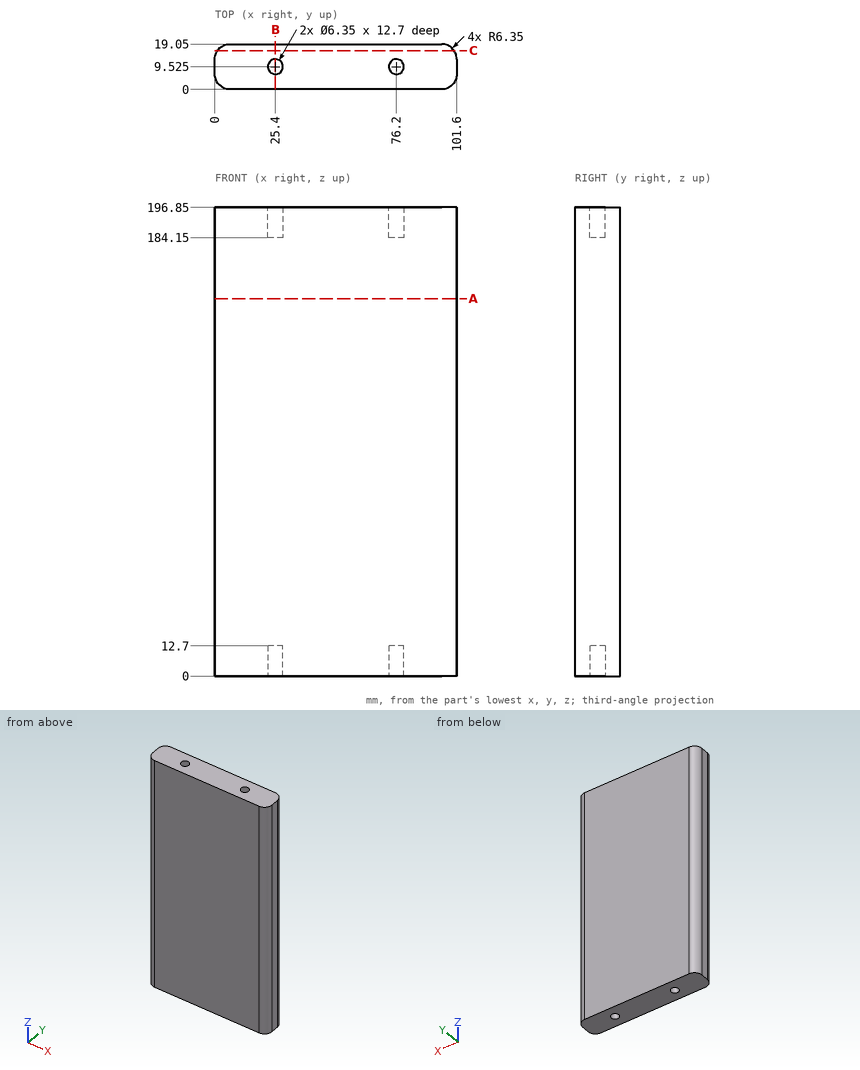
Verification items for this drawing (mm, ordinates from the low corner). Give positions to 0.01 mm unless a question says otherwise; leave off trailing zeros. Write each loop counter-clockwise with the first axis right and the second up, starting at its lowest first coordinate (ties: lowest second). Pieces come first, ordered by that corner, then holes. Notation, with made-up numbers: (-40, 69.5) - (2, 69.5) arc R24 ccw to (2, 91.5) - close; hole circle Ø8 at (51.25, 53). An arc over 180 degrees is marked (long way). Answer as a JSON object with one key per item and string values. Group by question number.
1) Depth check by flat-ended pin: P1, Ø5, axis at x = 76.2, y = 9.525, coming from the +Z side; P2, Ø1.5, axis at y = 15, z = 123, coming from the +X side; P3, Ø3, axis at y = 2.5, z = 138.5, coming from the -X side. Enter the tip coordinate at first touch or a pass-through.
2) Sectioned sample at C-C (y = 16.25). Record the cut outline in (x, z).
3) Thickness scan on probe 1 along Y at (x, z) = (25, 187); probe 2 along X at (y, z) = (7.25, 187); probe 3 along Z at (x, y) = (26, 8.25). Record the ranges inside material, lowest first. Write a range as from..to.
4) Sectioned sample at B-B (x = 25.4). Record the cut outline in (y, z).
5) Sectioned sample at A-A (z = 158.5). Record the cut outline in (x, y).
Geometry results:
{
 "1": {"P1": "stops at z = 184.15", "P2": "stops at x = 101.41", "P3": "stops at x = 0.45"},
 "2": {"outline": "(1.09, 0) - (100.51, 0) - (100.51, 196.85) - (1.09, 196.85) - close"},
 "3": {"probe 1": "y = 0..6.38, 12.67..19.05", "probe 2": "x = 0..23.19, 27.61..73.99, 78.41..101.6", "probe 3": "z = 12.7..184.15"},
 "4": {"outline": "(0, 0) - (6.35, 0) - (6.35, 12.7) - (12.7, 12.7) - (12.7, 0) - (19.05, 0) - (19.05, 196.85) - (12.7, 196.85) - (12.7, 184.15) - (6.35, 184.15) - (6.35, 196.85) - (0, 196.85) - close"},
 "5": {"outline": "(0, 6.35) arc R6.35 ccw to (6.35, 0) - (95.25, 0) arc R6.35 ccw to (101.6, 6.35) - (101.6, 12.7) arc R6.35 ccw to (95.25, 19.05) - (6.35, 19.05) arc R6.35 ccw to (0, 12.7) - close"}
}
